Input: part model. Units: mm. Frame: model coordinates. A direction names the side the tool comes from. Give positions to 0.01 mm unless a question says otherwise; leave off trailing zeros. Loops run counter-clockwise (first coordinate to the right, second up) from the corner with the lowest first, then second, coordinate; pieces in that order, holes last. Notation, with made-up numbers: M 4,-2 L 22,-2 A27 ccw 22,25 Z; hole C 17,67.25 d9. An arc over 180 degrees is marked long. Answer as a JSON object with one key per item and string values. Group by question number.
```python
from build123d import *

# Parameters (mm, degrees)
SKETCH2_W = 8.73125
SKETCH2_H = 0.81407
SKETCH3_W = 8.73125
SKETCH3_H = 0.37084


with BuildPart() as part:
    # Sketch1 → BODY (revolve)
    with BuildSketch(Plane.XY, mode=Mode.PRIVATE) as body_sk:
        Polygon((7.14375, 14.2875), (7.14375, 13.49375), (7.9375, 12.7), (7.9375, 3.175), (7.14375, 2.38125), (8.73125, 0.79375), (8.73125, 0), (0, 0), (0, 14.2875), align=None)
    revolve(body_sk.sketch.rotate(Axis((0, 17.35888354, 0), (0, -1, 0)), 90), axis=Axis((0, 17.35888354, 0), (0, -1, 0)))

    # Sketch6 → BORE-1 (revolve, cut)
    with BuildSketch(Plane.XY, mode=Mode.PRIVATE) as bore_1_sk:
        Polygon((0, 13.49375), (1.26746, 12.761981628), (1.26746, 12.444481628), (1.58496, 12.444481628), (1.58496, 0.635), (2.21996, 0), (0, 0), align=None)
    revolve(bore_1_sk.sketch.rotate(Axis((0, 13.952718453, 0), (0, -1, 0)), 90), axis=Axis((0, 13.952718453, 0), (0, -1, 0)), mode=Mode.SUBTRACT)

    # Sketch2 → SET SCREW (revolve, cut)
    with BuildSketch(Plane.XY, mode=Mode.PRIVATE) as set_screw_sk:
        with Locations((4.365625, 6.757035)):
            Rectangle(SKETCH2_W, SKETCH2_H)
    revolve(set_screw_sk.sketch.rotate(Axis((-2.248807984, 6.35, 0), (1, 0, 0)), 90), axis=Axis((-2.248807984, 6.35, 0), (1, 0, 0)), mode=Mode.SUBTRACT)

    # Sketch3 → SUB DRILL (revolve, cut)
    with BuildSketch(Plane(origin=(0, 0, 0), x_dir=(0, 0, -1), z_dir=(1, 0, 0)), mode=Mode.PRIVATE) as sub_drill_sk:
        with Locations((4.365625, 6.53542)):
            Rectangle(SKETCH3_W, SKETCH3_H)
    revolve(sub_drill_sk.sketch.rotate(Axis((0, 6.35, 0), (0, 0, -1)), 90), axis=Axis((0, 6.35, 0), (0, 0, -1)), mode=Mode.SUBTRACT)


solid = part.part
```
1. First-contact query: P1, Ø3.5, axis at x = 0, z = 0, coming from the -Y side; P2, Ø5, axis at y = 9, z = -1.5, coming from the -X side; P3, Ø2, axis at y = 2.5, z = 5, coming from the +X side. Flat tips, straight axial feed; report the tip coordinate or a pass-through.
2. Reachability of faces 1 (the cylindrical face through (-0.38, 12.6, 1.21)), 2 (the cylindrical face through (4.69, 7.07, 0.38)), 3 (the cylindrical face through (-0.314, 13.885, -7.137)) from +Z, -Z, +X, -X, +Y, -Y: full face, straight path, thin tool, end or side. Return the list, or none.
3. Mould query, pull axis X, two halves, no side actions, for faces 4 (the cylindrical face through (8.524, 0.391, -1.893)), 5 (the flat face through (0, 14.288, 0)), 6 (the cylindrical face through (-1.34, 6.46, 0.85)). Classes: pulls with the +X half, pulls with the -X half, needs draft (parallel to the pull), parting line crosses it, or undercut.
4. Material intervals for L1, parallel to Y at x = 5.25, z = 0; L2, parallel to Y at x = 0, z = -6.25; L3, parallel to X at y = 9, z = 0, sorted ascending.
5. Section A-A (y = 6.35). Output: boundary loops of the cut face in (x, z) (1 decimal).
6. Section B-B (y = 8.5). Output: boundary loops of the cut face in (x, z) (1 decimal), then the cut area to 3 significant figures.
Geometry results:
{
 "1": {"P1": "y = 0.47", "P2": "x = -7.94", "P3": "x = 6.7"},
 "2": {"face 1": "-Y", "face 2": "+X", "face 3": "+Y"},
 "3": {"face 4": "parting line crosses it", "face 5": "needs draft", "face 6": "undercut"},
 "4": {"L1": "0 to 5.54, 7.16 to 14.29", "L2": "0 to 5.98, 6.72 to 14.29", "L3": "-7.94 to -1.58, 1.58 to 7.94"},
 "5": {"outline": "M -0.4,-7.9 L -0.4,-1.5 A1.6 cw long 1.4,0.8 L 7.9,0.8 A7.9 ccw long Z; M 0.4,-7.9 A7.9 ccw 7.9,-0.8 L 1.4,-0.8 A1.6 cw 0.4,-1.5 Z"},
 "6": {"outline": "C 0,0 d15.9; hole C 0,0 d3.2", "area": "190 mm2"}
}
